```python
from build123d import *

# Parameters (mm, degrees)
SKETCH1_R           = 14.6939
BOSS_EXTRUDE1_DEPTH = 101.6
SKETCH2_R           = 20.32
BOSS_EXTRUDE2_DEPTH = 35.56
SKETCH3_R           = 10.7442
BOSS_EXTRUDE3_DEPTH = 45.72
CUT_EXTRUDE1_DEPTH  = 14.1986


with BuildPart() as part:
    # Sketch1 → Boss-Extrude1 (new body)
    with BuildSketch(Plane.XY):
        Circle(SKETCH1_R)
    extrude(amount=BOSS_EXTRUDE1_DEPTH)

    # Sketch2 → Boss-Extrude2 (add)
    with BuildSketch(Plane(origin=(0, 0, 0), x_dir=(-1, 0, 0), z_dir=(0, 0, -1))):
        Circle(SKETCH2_R)
    extrude(amount=BOSS_EXTRUDE2_DEPTH)

    # Sketch3 → Boss-Extrude3 (add)
    with BuildSketch(Plane(origin=(0, 0, -35.56), x_dir=(-1, 0, 0), z_dir=(0, 0, -1))):
        Circle(SKETCH3_R)
    extrude(amount=BOSS_EXTRUDE3_DEPTH)

    # Sketch5 → Cut-Extrude1 (cut)
    with BuildSketch(Plane.XY):
        with BuildLine():
            ThreePointArc((-9.602914805, 11.121813002), (0, 14.6939), (9.602914805, 11.121813002))
            Line((9.602914805, 11.121813002), (12.018168226, 13.919088355))
            ThreePointArc((12.018168226, 13.919088355), (0, 18.3896), (-12.018168226, 13.919088355))
            Line((-12.018168226, 13.919088355), (-9.602914805, 11.121813002))
        make_face()
        with BuildLine():
            ThreePointArc((14.433229999, 2.755461671), (12.725290681, -7.34695), (4.830315193, -13.877274673))
            Line((4.830315193, -13.877274673), (6.0452, -17.367583169))
            ThreePointArc((6.0452, -17.367583169), (15.925860765, -9.1948), (18.063368226, 3.448494813))
            Line((18.063368226, 3.448494813), (14.433229999, 2.755461671))
        make_face()
        with BuildLine():
            Line((-6.0452, -17.367583169), (-4.830315193, -13.877274673))
            ThreePointArc((-4.830315193, -13.877274673), (-12.725290681, -7.34695), (-14.433229999, 2.755461671))
            Line((-14.433229999, 2.755461671), (-18.063368226, 3.448494813))
            ThreePointArc((-18.063368226, 3.448494813), (-15.925860765, -9.1948), (-6.0452, -17.367583169))
        make_face()
    extrude(amount=-CUT_EXTRUDE1_DEPTH, mode=Mode.SUBTRACT)


solid = part.part
```
Can you work these out from the model? Positions are in its coordinate system, mm. A direction names the side the tool comes from. Coordinates: 2 decimals unless noted, no trailing zeros. Order: outer loops, then holes, each group sorted by start corner. A loop starts at its lowest first (then second) coordinate and runs counter-clockwise, first axis right, second up. Notation, with made-up numbers: (-23, -23) - (-4, -23) arc R30 ccw to (-4, 9) - close; hole circle Ø1 at (81.25, 56). An arc over 180 degrees is marked (long way). Answer in a Markdown table with one row per item.
1. Suppose I cut it at C-C (z = 88.5). Please give me the cut outline in (x, y), and give its area (3 significant figures).
Reply:
| item | result |
|---|---|
| outline | circle Ø29.39 at (0, 0) |
| area | 678 mm^2 |
2. Suppose I cut it at B-B (y = 0). Please give me the cut outline in (x, z).
Reply:
| item | result |
|---|---|
| outline | (-20.32, -35.56) - (-10.74, -35.56) - (-10.74, -81.28) - (10.74, -81.28) - (10.74, -35.56) - (20.32, -35.56) - (20.32, 0) - (18.39, 0) - (18.39, -14.2) - (14.69, -14.2) - (14.69, 101.6) - (-14.69, 101.6) - (-14.69, -14.2) - (-18.39, -14.2) - (-18.39, 0) - (-20.32, 0) - close |
3. If I drill on line 1 along Z through (x, y) = (-8, 16); line 2 along X through (y, z) = (-16, -6); line 3 along Z through (x, y) = (8, -18), over which ranges is the centre line in solid material (lowest first)?
Reply:
| item | result |
|---|---|
| line 1 | z = -35.56 to -14.2 |
| line 2 | x = -12.53 to -9.07, -5.57 to 5.57, 9.07 to 12.53 |
| line 3 | z = -35.56 to 0 |
4. If we mould it in two halves opening along X, with no side actions, what happens to faces 4 (the flat face through (-16.223, 3.097, -7)), 5 (the cylindrical face through (15.833, -9.353, -7)), 6 (the cylindrical face through (2.33, -10.49, -58.1)), 7 (the flat face through (0, 0, 101.6))? For each: pulls with the +X half, pulls with the -X half, needs draft (parallel to the pull), parting line crosses it, or undercut.
Reply:
| item | result |
|---|---|
| face 4 | undercut |
| face 5 | undercut |
| face 6 | parting line crosses it |
| face 7 | needs draft |
5. For faces 1 (the flat face through (-9, -9, -35.56)), 2 (the flat face through (0, 0, -81.28)), 3 (the flat face through (0, 16, -14.199)), which set-ups out of +Z, -Z, +X, -X, +Y, -Y let a thin tool reach every point of the face, with its end or its side?
Reply:
| item | result |
|---|---|
| face 1 | -Z |
| face 2 | -Z, +X, -X, +Y, -Y |
| face 3 | +Z |
6. Suppose I cut it at A-A (x = 0). Please give me the cut outline in (y, z).
Reply:
| item | result |
|---|---|
| outline | (-20.32, -35.56) - (-10.74, -35.56) - (-10.74, -81.28) - (10.74, -81.28) - (10.74, -35.56) - (20.32, -35.56) - (20.32, 0) - (18.39, 0) - (18.39, -14.2) - (14.69, -14.2) - (14.69, 101.6) - (-14.69, 101.6) - (-14.69, 0) - (-20.32, 0) - close |
7. For pin 1 (6 mm diameter, centred on y = 2, z = 77, fed in from +X); pin 2 (8 mm diameter, centred on x = 4, y = 16, fed in from +Z); pin 3 (12 mm diameter, centred on x = -9, z = 48, fed in from +Y); pin 4 (3 mm diameter, centred on x = 1, z = 60, fed in from -Y), each with a flat end and sliding along its axis, tell me the tip position at first contact or that it passes through.
Reply:
| item | result |
|---|---|
| pin 1 | stops at x = 14.69 |
| pin 2 | stops at z = 101.6 |
| pin 3 | stops at y = 14.38 |
| pin 4 | stops at y = -14.69 |
8. Suppose I cut it at D-D (y = -8). Please give me the cut outline in (x, z).
Reply:
| item | result |
|---|---|
| outline | (-18.68, -35.56) - (-7.17, -35.56) - (-7.17, -81.28) - (7.17, -81.28) - (7.17, -35.56) - (18.68, -35.56) - (18.68, 0) - (16.56, 0) - (16.56, -14.2) - (12.33, -14.2) - (12.33, 101.6) - (-12.33, 101.6) - (-12.33, -14.2) - (-16.56, -14.2) - (-16.56, 0) - (-18.68, 0) - close |
